Input: part model. Units: mm. Frame: model coordinates. A direction names the side the tool comes from. Round coordinates to 2 decimals unless told otherwise and drop trailing zeros. Loops run counter-clockwise (first coordinate to the right, second up) from the corner with the lowest first, then second, coordinate; pieces in that order, holes last. Notation, with made-up numbers: (-32.5, 41) - (-10.5, 41) arc R23 cw to (-10.5, 53) - close; hole circle Ø5 at (-19, 63). An arc over 180 degrees is marked (long way). One line per question, with ' | ' between items. Start each with the question number.
from build123d import *

# Parameters (mm, degrees)
MOUNTING_PLATE_SKETCH_W        = 42
MOUNTING_PLATE_SKETCH_H        = 29
MOUNTING_PLATE_DEPTH           = 3
AXLE_COLLAR_CLEARANCE_SKETCH_R = 12.1
AXLE_COLLAR_CLEARANCE_DEPTH    = 3.2
M3_CAP_BOLT_HOLE_1_SKETCH_R    = 1.7
M3_CAP_BOLT_HOLE_1_DEPTH       = 3.2
M3_CAP_BOLT_HOLE_2_SKETCH_R    = 1.7
M3_CAP_BOLT_HOLE_2_DEPTH       = 3.2
CLAMP_SEAT_1_SKETCH_W          = 5
CLAMP_SEAT_1_SKETCH_H          = 8
CLAMP_SEAT_1_DEPTH             = 1.7
M2_SCREW_CLEARANCE_1_SKETCH_R  = 1.1
M2_SCREW_CLEARANCE_1_DEPTH     = 4.8
M2_INSERT_POCKET_1_SKETCH_R    = 1.6
M2_INSERT_POCKET_1_DEPTH       = 2.5
CLAMP_SEAT_2_SKETCH_W          = 5
CLAMP_SEAT_2_SKETCH_H          = 8
CLAMP_SEAT_2_DEPTH             = 1.7
M2_SCREW_CLEARANCE_2_SKETCH_R  = 1.1
M2_SCREW_CLEARANCE_2_DEPTH     = 4.8
M2_INSERT_POCKET_2_SKETCH_R    = 1.6
M2_INSERT_POCKET_2_DEPTH       = 2.5


with BuildPart() as part:
    # Mounting Plate Sketch → Mounting Plate (new body)
    with BuildSketch(Plane.XY):
        with Locations((0, -1.5)):
            Rectangle(MOUNTING_PLATE_SKETCH_W, MOUNTING_PLATE_SKETCH_H)
    extrude(amount=MOUNTING_PLATE_DEPTH)

    # Axle Collar Clearance Sketch → Axle Collar Clearance (cut)
    with BuildSketch(Plane.XY.offset(-0.1)):
        with Locations((0, -24)):
            Circle(AXLE_COLLAR_CLEARANCE_SKETCH_R)
    extrude(amount=AXLE_COLLAR_CLEARANCE_DEPTH, mode=Mode.SUBTRACT)

    # M3 Cap Bolt Hole 1 Sketch → M3 Cap Bolt Hole 1 (cut)
    with BuildSketch(Plane.XY.offset(-0.1)):
        with Locations((-12.515790027, -11.484209973)):
            Circle(M3_CAP_BOLT_HOLE_1_SKETCH_R)
    extrude(amount=M3_CAP_BOLT_HOLE_1_DEPTH, mode=Mode.SUBTRACT)

    # M3 Cap Bolt Hole 2 Sketch → M3 Cap Bolt Hole 2 (cut)
    with BuildSketch(Plane.XY.offset(-0.1)):
        with Locations((12.515790027, -11.484209973)):
            Circle(M3_CAP_BOLT_HOLE_2_SKETCH_R)
    extrude(amount=M3_CAP_BOLT_HOLE_2_DEPTH, mode=Mode.SUBTRACT)

    # Clamp Seat 1 Sketch → Clamp Seat 1 (add)
    with BuildSketch(Plane.XY.offset(2.9)):
        with Locations((-17, 0)):
            Rectangle(CLAMP_SEAT_1_SKETCH_W, CLAMP_SEAT_1_SKETCH_H)
    extrude(amount=CLAMP_SEAT_1_DEPTH)

    # M2 Screw Clearance 1 Sketch → M2 Screw Clearance 1 (cut)
    with BuildSketch(Plane.XY.offset(-0.1)):
        with Locations((-17, 0)):
            Circle(M2_SCREW_CLEARANCE_1_SKETCH_R)
    extrude(amount=M2_SCREW_CLEARANCE_1_DEPTH, mode=Mode.SUBTRACT)

    # M2 Insert Pocket 1 Sketch → M2 Insert Pocket 1 (cut)
    with BuildSketch(Plane.XY.offset(-0.1)):
        with Locations((-17, 0)):
            Circle(M2_INSERT_POCKET_1_SKETCH_R)
    extrude(amount=M2_INSERT_POCKET_1_DEPTH, mode=Mode.SUBTRACT)

    # Clamp Seat 2 Sketch → Clamp Seat 2 (add)
    with BuildSketch(Plane.XY.offset(2.9)):
        with Locations((17, 0)):
            Rectangle(CLAMP_SEAT_2_SKETCH_W, CLAMP_SEAT_2_SKETCH_H)
    extrude(amount=CLAMP_SEAT_2_DEPTH)

    # M2 Screw Clearance 2 Sketch → M2 Screw Clearance 2 (cut)
    with BuildSketch(Plane.XY.offset(-0.1)):
        with Locations((17, 0)):
            Circle(M2_SCREW_CLEARANCE_2_SKETCH_R)
    extrude(amount=M2_SCREW_CLEARANCE_2_DEPTH, mode=Mode.SUBTRACT)

    # M2 Insert Pocket 2 Sketch → M2 Insert Pocket 2 (cut)
    with BuildSketch(Plane.XY.offset(-0.1)):
        with Locations((17, 0)):
            Circle(M2_INSERT_POCKET_2_SKETCH_R)
    extrude(amount=M2_INSERT_POCKET_2_DEPTH, mode=Mode.SUBTRACT)


solid = part.part
(1) Section B-B, the plane x = -17. Output: boundary loops of the cut face in (y, z).
(2) Section D-D, the plane x = -12. Output: boundary loops of the cut face in (y, z).
(3) Section C-C, the plane z = 0.75. Output: boundary loops of the cut face in (x, y).
(4) Pull-direction query (Y, two-part tool) for faces 4 (the face through (16, 1, 4.6)), 5 (the face through (15.9, 0, 3.5)), 6 (the face through (0, 13, 1)); classes: released by +Y, released by -Y, zero draft, split by the parting line, or undercut.
(5) Section A-A, the plane y = 0. Output: boundary loops of the cut face in (x, z), plus the area to 3 significant figures.
(6) Line query: line 1 along X through (y, z) = (0, 0.85); line 2 along X through (y, z) = (0, 4.05); line 3 along Y through (x, z) = (-17, 3.05). Output: solid intervals per line, ascending. Write a range as from..to.
(7) Pin query (flat end, axial travel): P1, Ø6, axis at x = 4.5, y = 2, coming from the +Z side; P2, Ø0.8, axis at y = 1, z = 4, coming from the +X side; P3, Ø2.5, axis at x = 17, y = 0, coming from the -Z side. Return the tip coordinate at first contact, or that it passes through.
(8) Reachability of faces 1 (the face through (19.5, 0, 4)), 2 (the face through (-19.5, 0, 4)), 3 (the face through (17, 4, 4)) from +Z, -Z, +X, -X, +Y, -Y: full face, straight path, thin tool, end or side. Return the list, or none.
Derived:
1) outline: (-16, 0) - (-1.6, 0) - (-1.6, 2.4) - (-1.1, 2.4) - (-1.1, 4.6) - (-4, 4.6) - (-4, 3) - (-16, 3) - close; (1.1, 2.4) - (1.6, 2.4) - (1.6, 0) - (13, 0) - (13, 3) - (4, 3) - (4, 4.6) - (1.1, 4.6) - close
2) outline: (-16, 0) - (-13.1, 0) - (-13.1, 3) - (-16, 3) - close; (-9.86, 0) - (13, 0) - (13, 3) - (-9.86, 3) - close
3) outline: (-21, -16) - (-9.08, -16) arc R12.1 cw to (9.08, -16) - (21, -16) - (21, 13) - (-21, 13) - close; hole circle Ø3.2 at (-17, 0); hole circle Ø3.4 at (-12.52, -11.48); hole circle Ø3.4 at (12.52, -11.48); hole circle Ø3.2 at (17, 0)
4) face 4: zero draft | face 5: undercut | face 6: released by +Y
5) outline: (-21, 0) - (-18.6, 0) - (-18.6, 2.4) - (-18.1, 2.4) - (-18.1, 4.6) - (-19.5, 4.6) - (-19.5, 3) - (-21, 3) - close; (-15.9, 2.4) - (-15.4, 2.4) - (-15.4, 0) - (15.4, 0) - (15.4, 2.4) - (15.9, 2.4) - (15.9, 4.6) - (14.5, 4.6) - (14.5, 3) - (-14.5, 3) - (-14.5, 4.6) - (-15.9, 4.6) - close; (18.1, 2.4) - (18.6, 2.4) - (18.6, 0) - (21, 0) - (21, 3) - (19.5, 3) - (19.5, 4.6) - (18.1, 4.6) - close | area: 117 mm²
6) line 1: x = -21..-18.6, -15.4..15.4, 18.6..21 | line 2: x = -19.5..-18.1, -15.9..-14.5, 14.5..15.9, 18.1..19.5 | line 3: y = -4..-1.1, 1.1..4
7) P1: stops at z = 3 | P2: stops at x = 19.5 | P3: stops at z = 2.4
8) face 1: +Z, +X, +Y, -Y | face 2: +Z, -X, +Y, -Y | face 3: +Z, +X, -X, +Y
